from build123d import *

# Parameters (mm, degrees)
F0_R     = 2.38125
F1_DEPTH = 3.175


with BuildPart() as f1:
    # F0 (on Right) → F1 (new body)
    with BuildSketch(Plane.YZ):
        with BuildLine():
            Line((155.575, 9.525), (0, 9.525))
            ThreePointArc((0, 9.525), (-9.525, 0), (0, -9.525))
            Line((0, -9.525), (155.575, -9.525))
            ThreePointArc((155.575, -9.525), (165.1, 0), (155.575, 9.525))
        make_face()
        Circle(F0_R, mode=Mode.SUBTRACT)
        with Locations((155.575, 0)):
            Circle(F0_R, mode=Mode.SUBTRACT)
    extrude(amount=F1_DEPTH)


solid = f1.part
Could you check a few things on this model? Use its own coordinates, in mm. Round coordinates to 2 decimals unless told otherwise and drop trailing zeros. Order: outer loops, then holes, each group sorted by start corner. A loop starts at its lowest first (then second) coordinate and runs counter-clockwise, first axis right, second up.
Q1. Imagine slicing it at A-A, the plane z = 0. List the corners of the cut face in (x, y) for me (3 decimals).
Geometry says:
outline: (0, -9.525) - (3.175, -9.525) - (3.175, -2.381) - (0, -2.381) - close; (0, 2.381) - (3.175, 2.381) - (3.175, 153.194) - (0, 153.194) - close; (0, 157.956) - (3.175, 157.956) - (3.175, 165.1) - (0, 165.1) - close
Q2. Please list where these lines run through material, in increasing order: probe 1 along Y at (x, z) = (2.15, 0.5); probe 2 along Y at (x, z) = (2.95, 5.75); probe 3 along Y at (x, z) = (2.65, 4.25).
Geometry says:
probe 1: y = -9.51 to -2.33, 2.33 to 153.25, 157.9 to 165.09
probe 2: y = -7.59 to 163.17
probe 3: y = -8.52 to 164.1
Q3. Imagine slicing it at B-B, the plane x = 1.1. State how many separate pieces and enclosed holes the cut face has, then the cut area to 3 significant figures.
Geometry says:
separate pieces: 1
enclosed holes: 2
area: 3,210 mm2
Q4. I'm going to push flat-ended pins straight in: P1, Ø6, axis at y = 104.5, z = 0, coming from the -X side; P2, Ø1.5, axis at x = 0.5, z = 1, coming from the -Y side. Where does each tip first touch, or does it pass through?
Geometry says:
P1: stops at x = 0
P2: stops at y = -9.52
